```python
from build123d import *

# Parameters (mm, degrees)
SKETCH_1_W          = 110
SKETCH_1_H          = 270.99984649
SKETCH_1_R          = 2.1
EXTRUDE_1_DEPTH     = 4
CHAMFER_1_SIZE      = 10
CUT_EXTRUDE_1_DEPTH = 4
FILLET_1_R          = 5
EXTRUDE_2_DEPTH     = 4
CHAMFER_2_SIZE      = 10
FILLET_2_R          = 4
FILLET_3_R          = 5
SKETCH_5_R          = 1.6
CUT_EXTRUDE_2_DEPTH = 4
SKETCH_7_W          = 70
SKETCH_7_H          = 140
EXTRUDE_3_DEPTH     = 4
FILLET_4_R          = 6
SKETCH_8_R          = 2.1
CUT_EXTRUDE_3_DEPTH = 4
SKETCH_9_R          = 1.6
CUT_EXTRUDE_4_DEPTH = 4
CHAMFER_3_SIZE      = 5
SKETCH_11_W         = 114
SKETCH_11_H         = 114.028365308
CUT_EXTRUDE_5_DEPTH = 10
FILLET_5_R          = 3


with BuildPart() as part:
    # 草图1 → 凸台-拉伸1 (new body)
    with BuildSketch(Plane(origin=(0, 0, 0), x_dir=(1, 0, 0), z_dir=(0, 1, 0))):
        Rectangle(SKETCH_1_W, SKETCH_1_H)
        with Locations(Location((-35, 127.499923245, 0), (0, 0, 270))):
            Circle(SKETCH_1_R, mode=Mode.SUBTRACT)
        with Locations(Location((-20, 118.499923245, 0), (0, 0, 270))):
            Circle(SKETCH_1_R, mode=Mode.SUBTRACT)
        with Locations(Location((20, 118.499923245, 0), (0, 0, 270))):
            Circle(SKETCH_1_R, mode=Mode.SUBTRACT)
        with Locations(Location((35, 127.499923245, 0), (0, 0, 270))):
            Circle(SKETCH_1_R, mode=Mode.SUBTRACT)
        with Locations(Location((20, 102.499923245, 0), (0, 0, 270))):
            Circle(SKETCH_1_R, mode=Mode.SUBTRACT)
        with Locations(Location((35, 93.499923245, 0), (0, 0, 270))):
            Circle(SKETCH_1_R, mode=Mode.SUBTRACT)
        with Locations(Location((-35, 93.499923245, 0), (0, 0, 270))):
            Circle(SKETCH_1_R, mode=Mode.SUBTRACT)
        with Locations(Location((-20, 102.499923245, 0), (0, 0, 270))):
            Circle(SKETCH_1_R, mode=Mode.SUBTRACT)
        with Locations(Location((-35, -127.499923245, 0), (0, 0, 270))):
            Circle(SKETCH_1_R, mode=Mode.SUBTRACT)
        with Locations(Location((-20, -118.499923245, 0), (0, 0, 270))):
            Circle(SKETCH_1_R, mode=Mode.SUBTRACT)
        with Locations(Location((-20, -102.499923245, 0), (0, 0, 270))):
            Circle(SKETCH_1_R, mode=Mode.SUBTRACT)
        with Locations(Location((20, -118.499923245, 0), (0, 0, 270))):
            Circle(SKETCH_1_R, mode=Mode.SUBTRACT)
        with Locations(Location((20, -102.499923245, 0), (0, 0, 270))):
            Circle(SKETCH_1_R, mode=Mode.SUBTRACT)
        with Locations(Location((35, -93.499923245, 0), (0, 0, 270))):
            Circle(SKETCH_1_R, mode=Mode.SUBTRACT)
        with Locations(Location((35, -127.499923245, 0), (0, 0, 270))):
            Circle(SKETCH_1_R, mode=Mode.SUBTRACT)
    extrude(amount=EXTRUDE_1_DEPTH)

    # 倒角1
    chamfer_1_edges = [part.edges().sort_by_distance(p)[0] for p in [
        (55, 2, -135.499923245),
        (55, 2, 135.499923245),
        (-55, 2, 135.499923245),
        (-55, 2, -135.499923245),
    ]]
    chamfer(chamfer_1_edges, length=CHAMFER_1_SIZE)

    # 草图2 → 切除-拉伸1 (cut)
    with BuildSketch(Plane(origin=(0, 4, 0), x_dir=(1, 0, 0), z_dir=(0, 1, 0))):
        Polygon((-25, 45), (-40, 30), (-40, -30), (-25, -45), (-25, -65), (25, -65), (25, -45), (40, -30), (40, 30), (25, 45), (25, 65), (-25, 65), align=None)
    extrude(amount=-CUT_EXTRUDE_1_DEPTH, mode=Mode.SUBTRACT)

    # 圆角1
    fillet_1_edges = [part.edges().sort_by_distance(p)[0] for p in [
        (25, 2, -65),
        (25, 2, 65),
        (-25, 2, 65),
        (-25, 2, -65),
    ]]
    fillet(fillet_1_edges, radius=FILLET_1_R)

    # 草图3 → 凸台-拉伸2 (add)
    with BuildSketch(Plane(origin=(0, 4, 0), x_dir=(1, 0, 0), z_dir=(0, 1, 0))):
        Polygon((55, 110.499923245), (85, 110.499923245), (85, 93.499923245), (85, -102.499923245), (85, -110.499923245), (55, -110.499923245), (55, -102.499923245), (55, 93.499923245), align=None)
        Polygon((-85, 93.499923245), (-85, -102.499923245), (-85, -110.499923245), (-55, -110.499923245), (-55, -102.499923245), (-55, 93.499923245), (-55, 110.499923245), (-85, 110.499923245), align=None)
    extrude(amount=-EXTRUDE_2_DEPTH)

    # 倒角2
    chamfer_2_edges = [part.edges().sort_by_distance(p)[0] for p in [
        (-85, 2, -110.499923245),
        (-85, 2, 110.499923245),
        (85, 2, 110.499923245),
        (85, 2, -110.499923245),
    ]]
    chamfer(chamfer_2_edges, length=CHAMFER_2_SIZE)

    # 圆角2
    fillet_2_edges = [part.edges().sort_by_distance(p)[0] for p in [
        (-55, 2, -110.499923245),
        (55, 2, -110.499923245),
        (55, 2, 110.499923245),
        (-55, 2, 110.499923245),
    ]]
    fillet(fillet_2_edges, radius=FILLET_2_R)

    # 圆角3
    fillet_3_edges = [part.edges().sort_by_distance(p)[0] for p in [
        (40, 2, -30),
        (40, 2, 30),
        (-40, 2, 30),
        (-40, 2, -30),
    ]]
    fillet(fillet_3_edges, radius=FILLET_3_R)

    # 草图5 → 切除-拉伸2 (cut)
    with BuildSketch(Plane(origin=(0, 4, 0), x_dir=(1, 0, 0), z_dir=(0, 1, 0))):
        with Locations(Location((-65, 65, 0), (0, 0, 270))):
            Circle(SKETCH_5_R)
        with Locations(Location((65, 65, 0), (0, 0, 270))):
            Circle(SKETCH_5_R)
        with Locations(Location((65, -65, 0), (0, 0, 270))):
            Circle(SKETCH_5_R)
        with Locations(Location((-65, -65, 0), (0, 0, 270))):
            Circle(SKETCH_5_R)
    extrude(amount=-CUT_EXTRUDE_2_DEPTH, mode=Mode.SUBTRACT)

    # 草图7 → 凸台-拉伸3 (add)
    with BuildSketch(Plane(origin=(0, 4, 0), x_dir=(1, 0, 0), z_dir=(0, 1, 0))):
        Polygon((-85, 0), (-85, 70), (-155, 70), (-155, -70), (-85, -70), align=None)
        with Locations((120, 0)):
            Rectangle(SKETCH_7_W, SKETCH_7_H)
    extrude(amount=-EXTRUDE_3_DEPTH)

    # 圆角4
    fillet_4_edges = [part.edges().sort_by_distance(p)[0] for p in [
        (-85, 2, 70),
        (-85, 2, -70),
        (85, 2, 70),
        (85, 2, -70),
    ]]
    fillet(fillet_4_edges, radius=FILLET_4_R)

    # 草图8 → 切除-拉伸3 (cut)
    with BuildSketch(Plane(origin=(0, 4, 0), x_dir=(1, 0, 0), z_dir=(0, 1, 0))):
        with Locations(Location((105, 65, 0), (0, 0, 270))):
            Circle(SKETCH_8_R)
        with Locations(Location((145, 65, 0), (0, 0, 270))):
            Circle(SKETCH_8_R)
        with Locations(Location((145, 45, 0), (0, 0, 270))):
            Circle(SKETCH_8_R)
        with Locations(Location((105, 45, 0), (0, 0, 270))):
            Circle(SKETCH_8_R)
        with Locations(Location((145, -45, 0), (0, 0, 270))):
            Circle(SKETCH_8_R)
        with Locations(Location((145, -65, 0), (0, 0, 270))):
            Circle(SKETCH_8_R)
        with Locations(Location((105, -65, 0), (0, 0, 270))):
            Circle(SKETCH_8_R)
        with Locations(Location((105, -45, 0), (0, 0, 270))):
            Circle(SKETCH_8_R)
        with Locations(Location((-145, 65, 0), (0, 0, 270))):
            Circle(SKETCH_8_R)
        with Locations(Location((-105, 65, 0), (0, 0, 270))):
            Circle(SKETCH_8_R)
        with Locations(Location((-105, 45, 0), (0, 0, 270))):
            Circle(SKETCH_8_R)
        with Locations(Location((-145, 45, 0), (0, 0, 270))):
            Circle(SKETCH_8_R)
        with Locations(Location((-145, -45, 0), (0, 0, 270))):
            Circle(SKETCH_8_R)
        with Locations(Location((-105, -45, 0), (0, 0, 270))):
            Circle(SKETCH_8_R)
        with Locations(Location((-105, -65, 0), (0, 0, 270))):
            Circle(SKETCH_8_R)
        with Locations(Location((-145, -65, 0), (0, 0, 270))):
            Circle(SKETCH_8_R)
    extrude(amount=-CUT_EXTRUDE_3_DEPTH, mode=Mode.SUBTRACT)

    # 草图9 → 切除-拉伸4 (cut)
    with BuildSketch(Plane(origin=(0, 4, 0), x_dir=(1, 0, 0), z_dir=(0, 1, 0))):
        with Locations(Location((-135, 47.5, 0), (0, 0, 270))):
            Circle(SKETCH_9_R)
        with Locations(Location((-115, 47.5, 0), (0, 0, 90))):
            Circle(SKETCH_9_R)
        with Locations(Location((-115, -47.5, 0), (0, 0, 270))):
            Circle(SKETCH_9_R)
        with Locations(Location((-135, -47.5, 0), (0, 0, 90))):
            Circle(SKETCH_9_R)
        with Locations(Location((135, -47.5, 0), (0, 0, 270))):
            Circle(SKETCH_9_R)
        with Locations(Location((115, -47.5, 0), (0, 0, 90))):
            Circle(SKETCH_9_R)
        with Locations(Location((115, 47.5, 0), (0, 0, 270))):
            Circle(SKETCH_9_R)
        with Locations(Location((135, 47.5, 0), (0, 0, 90))):
            Circle(SKETCH_9_R)
        with BuildLine():
            Line((-130, 29.028690408), (-80, 29.028690408))
            ThreePointArc((-80, 29.028690408), (-76, 25.028690408), (-80, 21.028690408))
            Line((-80, 21.028690408), (-130, 21.028690408))
            ThreePointArc((-130, 21.028690408), (-134, 25.028690408), (-130, 29.028690408))
        make_face()
        with BuildLine():
            Line((-130, 14.028690408), (-80, 14.028690408))
            ThreePointArc((-80, 14.028690408), (-76, 10.028690408), (-80, 6.028690408))
            Line((-80, 6.028690408), (-130, 6.028690408))
            ThreePointArc((-130, 6.028690408), (-134, 10.028690408), (-130, 14.028690408))
        make_face()
        with BuildLine():
            Line((-130, -29.028690408), (-80, -29.028690408))
            ThreePointArc((-80, -29.028690408), (-76, -25.028690408), (-80, -21.028690408))
            Line((-80, -21.028690408), (-130, -21.028690408))
            ThreePointArc((-130, -21.028690408), (-134, -25.028690408), (-130, -29.028690408))
        make_face()
        with BuildLine():
            Line((-130, -14.028690408), (-80, -14.028690408))
            ThreePointArc((-80, -14.028690408), (-76, -10.028690408), (-80, -6.028690408))
            Line((-80, -6.028690408), (-130, -6.028690408))
            ThreePointArc((-130, -6.028690408), (-134, -10.028690408), (-130, -14.028690408))
        make_face()
        with BuildLine():
            Line((130, 29.028690408), (80, 29.028690408))
            ThreePointArc((80, 29.028690408), (76, 25.028690408), (80, 21.028690408))
            Line((80, 21.028690408), (130, 21.028690408))
            ThreePointArc((130, 21.028690408), (134, 25.028690408), (130, 29.028690408))
        make_face()
        with BuildLine():
            Line((130, 14.028690408), (80, 14.028690408))
            ThreePointArc((80, 14.028690408), (76, 10.028690408), (80, 6.028690408))
            Line((80, 6.028690408), (130, 6.028690408))
            ThreePointArc((130, 6.028690408), (134, 10.028690408), (130, 14.028690408))
        make_face()
        with BuildLine():
            Line((130, -29.028690408), (80, -29.028690408))
            ThreePointArc((80, -29.028690408), (76, -25.028690408), (80, -21.028690408))
            Line((80, -21.028690408), (130, -21.028690408))
            ThreePointArc((130, -21.028690408), (134, -25.028690408), (130, -29.028690408))
        make_face()
        with BuildLine():
            Line((130, -14.028690408), (80, -14.028690408))
            ThreePointArc((80, -14.028690408), (76, -10.028690408), (80, -6.028690408))
            Line((80, -6.028690408), (130, -6.028690408))
            ThreePointArc((130, -6.028690408), (134, -10.028690408), (130, -14.028690408))
        make_face()
    extrude(amount=-CUT_EXTRUDE_4_DEPTH, mode=Mode.SUBTRACT)

    # 倒角3
    chamfer_3_edges = [part.edges().sort_by_distance(p)[0] for p in [
        (155, 2, -70),
        (155, 2, 70),
        (-155, 2, 70),
        (-155, 2, -70),
    ]]
    chamfer(chamfer_3_edges, length=CHAMFER_3_SIZE)

    # 草图11 → 切除-拉伸5 (cut)
    with BuildSketch(Plane(origin=(0, 4, 0), x_dir=(1, 0, 0), z_dir=(0, 1, 0))):
        Rectangle(SKETCH_11_W, SKETCH_11_H)
    extrude(amount=-CUT_EXTRUDE_5_DEPTH, mode=Mode.SUBTRACT)

    # 圆角5
    fillet_5_edges = [part.edges().sort_by_distance(p)[0] for p in [
        (-57, 2, 57.014182654),
        (57, 2, -57.014182654),
        (57, 2, 57.014182654),
        (-57, 2, -57.014182654),
    ]]
    fillet(fillet_5_edges, radius=FILLET_5_R)


solid = part.part
```
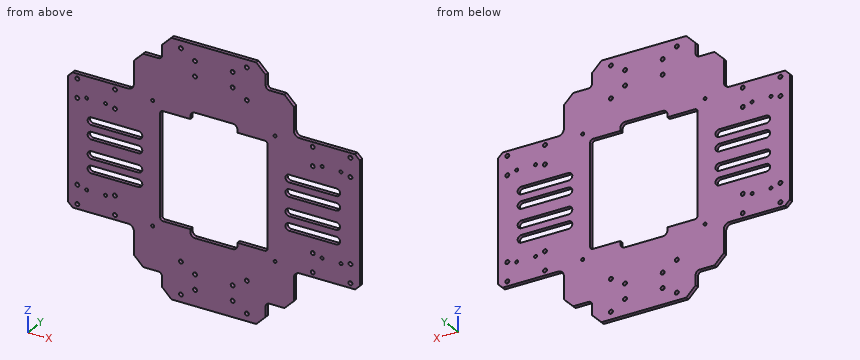
The model under review builds one solid part; all positions refer to its coordinate system, in mm. Coordinates: 2 decimals unless noted, no trailing zeros. One line per item, written item: value. Start each with the question number.
Q1. Clearance check with flat-ended pins moving along their axes: P1, Ø2, axis at y = 1, z = 92.5, coming from the -X side; P2, Ø2, axis at x = 133.5, y = 2, coming from the -Z side; P3, Ø1.2, axis at y = 1, z = 118, coming from the -X side. State where each tip first meets the part, or that it passes through.
Q2. To check wall thickness, follow probe 1 along Z at (x, y) = (96, 1.65); probe 2 along X at (y, z) = (3.1, -47.5); probe 3 along X at (y, z) = (2.05, -118.5). State the ranges of each line that lie inside material, in increasing order.
Q3. Add section A-A, the plane y = 1.5. Count the separate pieces of the cut face and the enclosed holes in it, then the cut area to 3 significant figures.
Response:
1. P1: x = -85
1. P2: z = -70
1. P3: x = -55
2. probe 1: -70 to -29.03, -21.03 to -14.03, -6.03 to 6.03, 14.03 to 21.03, 29.03 to 70
2. probe 2: -155 to -136.6, -133.4 to -116.6, -113.4 to -57, 57 to 113.4, 116.6 to 133.4, 136.6 to 155
2. probe 3: -55 to -22.1, -17.9 to 17.9, 22.1 to 55
3. separate pieces: 1
3. enclosed holes: 52
3. area: 44,400 mm²
